CAD build for the part. Positions are in the model's coordinates, mm. Face numbers are marked on the shaded views. A direction names the side the tool comes from. Round coordinates to 2 decimals unless told otherwise and drop trailing zeros. Order: outer loops, then holes, each group sorted by start corner. A loop starts at its lowest first (then second) coordinate and runs counter-clockwise, first axis right, second up. Notation, with made-up numbers: (25.25, -35) -> (73.25, -35) arc R34 cw to (73.25, 3) -> close; hole circle Ø9 at (71, 85). An arc over 180 degrees is marked (long way). Return JSON: item names as keys, results as strings. Group by question number.
Q1. Flat gauge pins, fed straight in: pin 1 (5 mm diameter, centred on x = 44, z = 18, fed in from +Y); pin 2 (6 mm diameter, centred on x = 39, y = -28, fed in from +Z); pin 3 (12 mm diameter, centred on x = 35.5, y = -12.5, fed in from -Z). Where does each tip first touch, or does it go through?
Q2. Which spindle directions (+Z, -Z, +X, -X, +Y, -Y) get a long thin tool onto all of the face, cutting with end or side? Do the marked faces 5, 6 and 7. Say none if no direction does.
Q3. Probe line 1 along X through (y, z) = (-3.5, 4); line 2 along Z through (x, y) = (30, -15); line 3 along X through (y, z) = (-15.5, 44.5). List the from-to ranges inside material, lowest first.
Q4. Cut at C-C (y = -32.5). Write the cut outline in (x, z).
Q5. Mould opens along X. For the marked faces 1, 2, 3 and 4 say: +X half, -X half, draft (parallel to the pull), parting line (faces both ways), or undercut.
Q6. Cut at A-A (y = -9). Write the cut outline in (x, z), then the cut area to 3 significant figures.
Q7. Cut at B-B (x = 30). Write the cut outline in (y, z), then the cut area to 3 significant figures.
Q8. Cut at D-D (z = 55). Write the cut outline in (x, y).
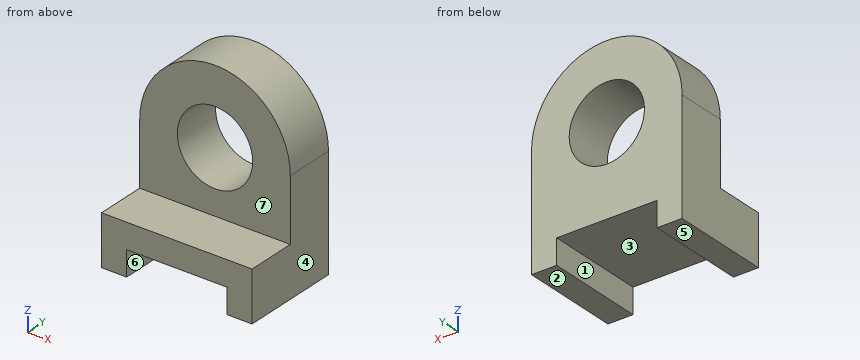
from build123d import *

# Parameters (mm, degrees)
F1_DEPTH = 40
F0_R     = 15
F2_DEPTH = 20


with BuildPart() as f1:
    # F0 (on Front) → F1 (new body)
    with BuildSketch(Plane.XZ):
        Polygon((0, 20), (0, 0), (10, 0), (10, 10), (50, 10), (50, 0), (60, 0), (60, 20), align=None)
    extrude(amount=F1_DEPTH)

    # F0 (on Front) → F2 (join)
    with BuildSketch(Plane.XZ):
        with BuildLine():
            Line((0, 45), (0, 20))
            Line((0, 20), (60, 20))
            Line((60, 20), (60, 45))
            ThreePointArc((60, 45), (30, 75), (0, 45))
        make_face()
        with Locations((30, 45)):
            Circle(F0_R, mode=Mode.SUBTRACT)
    extrude(amount=F2_DEPTH)


solid = f1.part
Solution:
{
 "1": {"pin 1": "stops at y = 0", "pin 2": "stops at z = 20", "pin 3": "stops at z = 10"},
 "2": {"face 5": "-Z, +X, -X, +Y, -Y", "face 6": "-Z, +Y, -Y", "face 7": "+Z, +X, -X, -Y"},
 "3": {"line 1": "x = 0 to 10, 50 to 60", "line 2": "z = 10 to 30, 60 to 75", "line 3": "x = 0 to 15.01, 44.99 to 60"},
 "4": {"outline": "(0, 0) -> (10, 0) -> (10, 10) -> (50, 10) -> (50, 0) -> (60, 0) -> (60, 20) -> (0, 20) -> close"},
 "5": {"face 1": "undercut", "face 2": "draft", "face 3": "undercut", "face 4": "+X half"},
 "6": {"outline": "(0, 0) -> (10, 0) -> (10, 10) -> (50, 10) -> (50, 0) -> (60, 0) -> (60, 45) arc R30 ccw to (0, 45) -> close; hole circle Ø30 at (30, 45)", "area": "3,010 mm²"},
 "7": {"outline": "(-40, 10) -> (0, 10) -> (0, 30) -> (-20, 30) -> (-20, 20) -> (-40, 20) -> close; (-20, 60) -> (0, 60) -> (0, 75) -> (-20, 75) -> close", "area": "900 mm²"},
 "8": {"outline": "(1.72, -20) -> (18.82, -20) -> (18.82, 0) -> (1.72, 0) -> close; (41.18, -20) -> (58.28, -20) -> (58.28, 0) -> (41.18, 0) -> close"}
}
